from build123d import *

# Parameters (mm, degrees)
SKETCH1_W               = 40
SKETCH1_H               = 10
BOSS_EXTRUDE1_DEPTH     = 27
SKETCH4_R               = 2.15
CUT_EXTRUDE1_DEPTH      = 1
CUT_EXTRUDE1_DEPTH_BACK = 11
FILLET1_R               = 1
SKETCH5_R               = 2.75
CUT_EXTRUDE2_DEPTH      = 1
CUT_EXTRUDE2_DEPTH_BACK = 28


with BuildPart() as part:
    # Sketch1 → Boss-Extrude1 (new body)
    with BuildSketch(Plane(origin=(0, 0, 0), x_dir=(1, 0, 0), z_dir=(0, 1, 0))):
        with Locations((20, 5)):
            Rectangle(SKETCH1_W, SKETCH1_H)
    extrude(amount=BOSS_EXTRUDE1_DEPTH)

    # Sketch4 → Cut-Extrude1 (cut, two sides)
    with BuildSketch(Plane(origin=(0, 0, -10), x_dir=(-1, 0, 0), z_dir=(0, 0, -1))) as cut_extrude1_sk:
        with Locations((-35.5, 13.5)):
            Circle(SKETCH4_R)
        with Locations((-4.5, 13.5)):
            Circle(SKETCH4_R)
    extrude(amount=CUT_EXTRUDE1_DEPTH, mode=Mode.SUBTRACT)
    extrude(cut_extrude1_sk.sketch, amount=-CUT_EXTRUDE1_DEPTH_BACK, mode=Mode.SUBTRACT)

    # Fillet1
    fillet1_edges = [part.edges().sort_by_distance(p)[0] for p in [
        (0, 13.5, -10),
        (40, 13.5, -10),
        (40, 13.5, 0),
        (0, 13.5, 0),
    ]]
    fillet(fillet1_edges, radius=FILLET1_R)

    # Sketch5 → Cut-Extrude2 (cut, two sides)
    with BuildSketch(Plane(origin=(0, 27, 0), x_dir=(1, 0, 0), z_dir=(0, 1, 0))) as cut_extrude2_sk:
        with Locations((12, 5)):
            Circle(SKETCH5_R)
        with Locations((28, 5)):
            Circle(SKETCH5_R)
    extrude(amount=CUT_EXTRUDE2_DEPTH, mode=Mode.SUBTRACT)
    extrude(cut_extrude2_sk.sketch, amount=-CUT_EXTRUDE2_DEPTH_BACK, mode=Mode.SUBTRACT)


solid = part.part
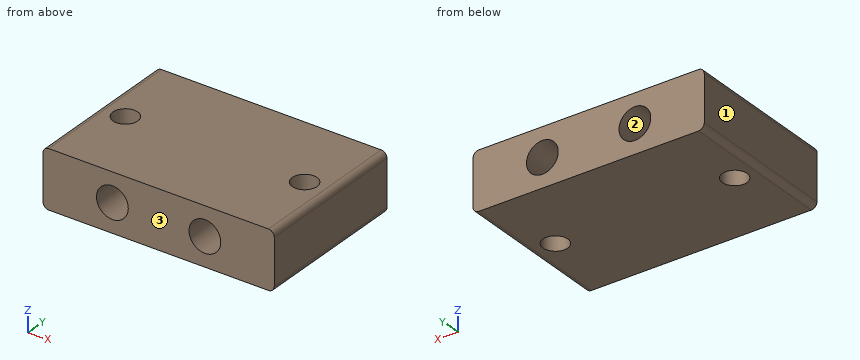
Check sheet for the modelled part. Datum: model origin and axes. Units: mm. Face numbers are marked on the shaded views. Give positions to 0.01 mm unless a question says otherwise; leave off trailing zeros. Loops run counter-clockwise (first coordinate to the right, second up) from the corner with the lowest first, then second, coordinate; pieces in that order, holes last. Notation, with made-up numbers: M 47.5,25.5 L 90.5,25.5 A11 ccw 90.5,29.5 Z; hole C -6.5,78 d6. An arc over 180 degrees is marked long. Use a Markdown table: item, result. Add a question column.
Q1. Scan lines: line 1 along Z through (x, y) = (28, 5.5); line 2 along X through (y, z) = (15.25, -4.75); line 3 along Y through (x, z) = (35.5, -6.25). Record each from-to range of solid material in increasing order. Write a range as [from, to].
Q2. Sectioned sample at A-A, the plane x = 35.5. Record the cut outline in (y, z), then the cut area to 3 significant figures.
Q3. Sectioned sample at C-C, the plane y = 2.5. Record the cut outline in (x, z), then the cut area to 3 significant figures.
Q4. Sectioned sample at D-D, the plane y = 13.5. Record the cut outline in (x, z).
Q5. Sectioned sample at B-B, the plane z = -5. Record the cut outline in (x, y).
Q6. Mould release check, pull along X, two halves, no side actions. Record for the marked faces 1, 2 and 3: pulls with the +X half, pulls with the -X half, needs draft (parallel to the pull), parting line crosses it, or undercut.
Q7. Go/stop test with a flat-tipped pin: pin 1 (6 mm diameter, centred on x = 17, z = -3, fed in from -Y). Record where the tip stops, or that it passes through.
Verdict:
| question | item | result |
|---|---|---|
| 1 | line 1 | [-10, -7.75], [-2.25, 0] |
| 1 | line 2 | [0, 3.25], [5.75, 9.26], [14.74, 25.26], [30.74, 34.25], [36.75, 40] |
| 1 | line 3 | [0, 11.35], [15.65, 27] |
| 2 | outline | M 0,-10 L 11.35,-10 L 11.35,0 L 0,0 Z; M 15.65,-10 L 27,-10 L 27,0 L 15.65,0 Z |
| 2 | area | 227 mm^2 |
| 3 | outline | M 0,-9 A1 ccw 1,-10 L 39,-10 A1 ccw 40,-9 L 40,-1 A1 ccw 39,0 L 1,0 A1 ccw 0,-1 Z; hole C 12,-5 d5.5; hole C 28,-5 d5.5 |
| 3 | area | 352 mm^2 |
| 4 | outline | M 0,-9 A1 ccw 1,-10 L 2.35,-10 L 2.35,0 L 1,0 A1 ccw 0,-1 Z; M 6.65,-10 L 33.35,-10 L 33.35,0 L 6.65,0 Z; M 37.65,-10 L 39,-10 A1 ccw 40,-9 L 40,-1 A1 ccw 39,0 L 37.65,0 Z; hole C 12,-5 d5.5; hole C 28,-5 d5.5 |
| 5 | outline | M 0,0 L 9.25,0 L 9.25,27 L 0,27 Z; M 14.75,0 L 25.25,0 L 25.25,27 L 14.75,27 Z; M 30.75,0 L 40,0 L 40,27 L 30.75,27 Z; hole C 4.5,13.5 d4.3; hole C 35.5,13.5 d4.3 |
| 6 | face 1 | pulls with the -X half |
| 6 | face 2 | undercut |
| 6 | face 3 | needs draft |
| 7 | pin 1 | y = 0 |
